Can you work these out from the model? Positions are in its coordinate system, mm. A direction names the side the tool comes from. Round coordinates to 2 decimals unless told otherwise and drop trailing zeros. Order: outer loops, then holes, each group sorted by start corner. A loop starts at its lowest first (then second) coordinate and runs counter-clockwise, first axis right, second up. Notation, with made-up numbers: M 46,70.25 L 66,70.25 A31 cw 66,108.25 Z; hole C -8.5,-2.5 d6. An arc over 180 degrees is marked long. One line per question, with ' | ' between items.
```python
from build123d import *

# Parameters (mm, degrees)
BOSS_EXTRUDE1_DEPTH = 7
SKETCH3_W           = 50
SKETCH3_H           = 212.444289875
CUT_EXTRUDE2_DEPTH  = 8


with BuildPart() as part:
    # Sketch1 → Boss-Extrude1 (new body)
    with BuildSketch(Plane.XY):
        with BuildLine():
            Line((0, 0), (0, 250))
            Line((0, 250), (50, 300))
            Line((50, 300), (125, 300))
            ThreePointArc((125, 300), (175, 250), (225, 300))
            Line((225, 300), (300, 300))
            Line((300, 300), (350, 250))
            Line((350, 250), (350, 0))
            Line((350, 0), (300, -50))
            Line((300, -50), (225, -50))
            ThreePointArc((225, -50), (175, 0), (125, -50))
            Line((125, -50), (50, -50))
            Line((50, -50), (0, 0))
        make_face()
    extrude(amount=BOSS_EXTRUDE1_DEPTH)

    # Sketch3 → Cut-Extrude2 (cut, through all)
    with BuildSketch(Plane.XY.offset(7)):
        with Locations((175, 192.120840959)):
            Rectangle(SKETCH3_W, SKETCH3_H)
    extrude(amount=-CUT_EXTRUDE2_DEPTH, mode=Mode.SUBTRACT)


solid = part.part
```
(1) On a 3-axis mill with a long thin cutter (end or side, diameter ignored), from which of +Z, -Z, +X, -X, +Y, -Y can I reach the whole of each face in a straight line? I mean faces 4 (the cylindrical face through (131.517, 275.318, 3.451)), 5 (the flat face through (25, -25, 3)). Say none if no direction works.
Final values:
face 4: +Z, -Z, +Y | face 5: +Z, -Z, -X, -Y
(2) Thinking about a two-plate mould opening in X: for faces 1 (the flat face through (325, 275, 3)), 2 (the cylindrical face through (218.117, 274.683, 3.451)), 3 (the flat face through (139, 127, 7)), which applies, released by +X, released by -X, zero draft, split by the parting line, or undercut?
Final values:
face 1: released by +X | face 2: undercut | face 3: zero draft
(3) If we section it at A-A on z = 4: Please give me the cut outline in (x, y), plus the area to 3 significant figures.
Final values:
outline: M 0,0 L 50,-50 L 125,-50 A50 cw 225,-50 L 300,-50 L 350,0 L 350,250 L 300,300 L 225,300 A50 cw 200,256.7 L 200,85.9 L 150,85.9 L 150,256.7 A50 cw 125,300 L 50,300 L 0,250 Z | area: 101,000 mm^2
(4) If we section it at D-D on x = 175: Please give me the cut outline in (y, z), plus the area to 3 significant figures.
Final values:
outline: M 0,0 L 85.9,0 L 85.9,7 L 0,7 Z | area: 601 mm^2
(5) Will this pin go through, and if not, where does the flat tip stop? pin 1 Ø2 at (x, z) = (165.5, 4.5) entering from +Y.
Final values:
pin 1: y = 85.9
(6) If we section it at C-C on x = 29: Please give me the cut outline in (y, z), plus the area to 3 significant figures.
Final values:
outline: M -29,0 L 279,0 L 279,7 L -29,7 Z | area: 2,160 mm^2
(7) If we section it at B-B on y = -16: Please give me the cut outline in (x, z).
Final values:
outline: M 16,0 L 138.34,0 L 138.34,7 L 16,7 Z; M 211.66,0 L 334,0 L 334,7 L 211.66,7 Z
(8) Please list where these lines run through material, in increasing order: probe 1 along X at (y, z) = (181, 5.5); probe 2 along X at (y, z) = (-27, 2.5); probe 3 along Y at (x, z) = (168, 3.25). Write a range as [from, to].
Final values:
probe 1: [0, 150], [200, 350] | probe 2: [27, 130.6], [219.4, 323] | probe 3: [-0.49, 85.9]
